Verification items for the finished model (mm, model axes). A direction names the side the tool comes from. Coordinates: 2 decimals unless noted, no trailing zeros. Order: outer loops, then holes, each group sorted by start corner. A loop starts at its lowest first (then second) coordinate and runs counter-clockwise, first axis right, second up. Notation, with made-up numbers: (-23, 14.5) -> (28, 14.5) arc R19 cw to (28, 50.5) -> close; hole circle Ø6 at (-29.75, 62.25). An arc over 180 degrees is marked (long way). Answer as CSV lines item,"result".
Autodesk Inventor part; units mm, degrees
ref_plane "YZ Plane" through (0, 0, 0) normal (1, 0, 0) x (0, 1, 0)
ref_plane "XZ Plane" through (0, 0, 0) normal (0, 1, 0) x (-1, 0, 0)
ref_plane "XY Plane" through (0, 0, 0) normal (0, 0, 1) x (1, 0, 0)
sketch "Sketch1" plane through (0, 0, 0) normal (0, 1, 0) x (-1, 0, 0)
  line L0 (-25, -25) -> (25, -25)
  line L1 (25, -25) -> (25, 25)
  line L2 (25, 25) -> (-25, 25)
  line L3 (-25, 25) -> (-25, -25)
  point P0 (0, 0)
  dimension "d2" = 50
  dimension "d3" = 50
extrude "Extrusion1" add sketch "Sketch1" along normal blind 4
sketch "Sketch2" plane through (0, 4, 0) normal (0, 1, 0) x (1, 0, 0)
  line L0 (-25, 25) -> (-25, -25)
  line L1 (-25, -25) -> (25, -25)
  line L2 (25, -25) -> (25, 25)
  line L3 (25, 25) -> (-25, 25)
  line L4 (-25, -25) -> (25, -25)
  line L5 (0, -25) -> (0, 25)
  line L6 (25, 25) -> (-25, 25)
  line L7 (0, -25) -> (-1.5, -25)
  line L8 (-1.5, -25) -> (1.5, -25)
  line L9 (1.5, -25) -> (1.5, 25)
  line L10 (1.5, 25) -> (-1.5, 25)
  line L11 (-1.5, 25) -> (-1.5, -25)
  line L12 (1.5, 9.2284) -> (-1.5, 9.2284)
  line L13 (1.5, 9.2284) -> (-1.5, 9.2284)
  line L14 (-1.5, 9.2284) -> (-1.5, 25)
  line L15 (-1.5, 25) -> (1.5, 25)
  line L16 (1.5, 25) -> (1.5, 9.2284)
  point P0 (0, 0)
  point P1 (1.5, 25)
  dimension "d6" = 1.5
  dimension "d7" = 3
extrude "Extrusion2" add sketch "Sketch2" along normal blind 3 contours L3 L5 L12 L11 | L3 L9 L12 L5
sketch "Sketch3" plane through (0, 4, 0) normal (0, 1, 0) x (1, 0, 0)
  line L0 (1.5, 25) -> (1.5, 9.2284)
  line L1 (1.5, 9.2284) -> (-1.5, 9.2284)
  line L2 (-1.5, 9.2284) -> (-1.5, 25)
  line L3 (-1.5, 25) -> (-25, 25)
  line L4 (-25, 25) -> (-25, -25)
  line L5 (-25, -25) -> (25, -25)
  line L6 (25, -25) -> (25, 25)
  line L7 (25, 25) -> (1.5, 25)
  line L8 (11.5, 24.5) -> (11.5, 9.7)
  line L9 (-11.5, 9.7) -> (-11.5, 24.5)
  line L10 (25, 25) -> (1.5, 25)
  line L11 (25, 25) -> (11.5, 25)
  line L12 (11.5, 25) -> (11.5, 9.7)
  line L13 (11.5, 9.7) -> (25, 9.7)
  line L14 (25, 9.7) -> (25, 25)
  line L15 (-11.5, 9.7) -> (-25, 9.7)
  line L16 (-25, 9.7) -> (-25, 25)
  line L17 (-25, 25) -> (-11.5, 25)
  line L18 (-11.5, 25) -> (-11.5, 9.7)
  point P0 (0, 0)
extrude "Extrusion3" cut sketch "Sketch3" against normal blind 10 contours L7 L6 L13 L8 L12 | L18 L9 L15 L4 L3
sketch "Sketch4" plane through (0, 0, 0) normal (0, -1, 0) x (1, 0, 0)
  line L0 (-11.5, -9.7) -> (-11.5, -25)
  line L1 (11.5, -25) -> (-11.5, -25)
  line L2 (11.5, -25) -> (11.5, -9.7)
  line L3 (11.5, -9.7) -> (25, -9.7)
  line L4 (25, 25) -> (25, -9.7)
  line L5 (-25, 25) -> (25, 25)
  line L6 (-25, -9.7) -> (-25, 25)
  line L7 (-25, -9.7) -> (-11.5, -9.7)
  point P0 (0, 0)
extrude "Extrusion4" cut sketch "Sketch4" against normal blind 1
sketch "Sketch5" plane through (-25, 4, 25) normal (0, 0, 1) x (1, 0, 0)
  line L0 (0, -3) -> (50, -3)
  line L1 (50, -3) -> (50, 0)
  line L2 (0, 0) -> (50, 0)
  line L3 (0, -3) -> (0, 0)
  line L4 (0, 0) -> (50, 0)
  line L5 (0, 0) -> (50, 0)
  line L6 (50, 0) -> (50, 3)
  line L7 (50, 3) -> (0, 3)
  line L8 (0, 3) -> (0, 0)
  point P0 (25, -4)
  dimension "d14" = 3
extrude "Extrusion5" add sketch "Sketch5" against normal up to surface (34.7 mm away) contours L8 L7 L6 L2
sketch "Sketch6" plane through (11.5, 4, -9.7) normal (0, 0, -1) x (-1, 0, 0)
  line L0 (-13.5, -3) -> (0, -3)
  line L1 (0, 0) -> (0, -3)
  line L2 (10, 0) -> (0, 0)
  line L3 (10, 3) -> (10, 0)
  line L4 (10, 3) -> (-13.5, 3)
  line L5 (-13.5, -3) -> (-13.5, 3)
  line L6 (23, -3) -> (36.5, -3)
  line L7 (36.5, 3) -> (36.5, -3)
  line L8 (36.5, 3) -> (13, 3)
  line L9 (13, 0) -> (13, 3)
  line L10 (23, 0) -> (13, 0)
  line L11 (23, 0) -> (23, -3)
  line L12 (0, 0.5) -> (0, 11.5)
  line L13 (23, 11.5) -> (23, 0.5)
  line L14 (10, 0) -> (0, 0)
  line L15 (0, 11.5) -> (0, 0)
  line L16 (23, 11.5) -> (23, 0)
  line L17 (0, 0) -> (0, -3)
  line L18 (10, 3) -> (-13.5, 3)
  line L19 (0, 0) -> (10, 0)
  line L20 (10, 0) -> (10, 3)
  line L21 (10, 3) -> (0, 3)
  line L22 (0, 3) -> (0, 0)
  line L23 (13, 0) -> (13, 3)
  line L24 (23, 0) -> (23, -3)
  line L25 (13, 3) -> (23, 3)
  line L26 (23, 3) -> (23, 0)
  line L27 (23, 0) -> (13, 0)
  line L28 (13, 0) -> (13, 3)
  point P0 (11.5, -4)
  point P1 (23, 0.5)
  point P2 (0, 3)
extrude "Extrusion6" cut sketch "Sketch6" against normal blind 20 contours L15 L12 L4 L3 L2 | L10 L9 L8 L13 L16
sketch "Sketch7" plane through (11.5, 4, 10.3) normal (0, 0, -1) x (-1, 0, 0)
  arc A0 (0, 2.75) -> (10, 2.7503) centre (4.9999, 5.9206) ccw
  arc A1 (13, 2.75) -> (23, 2.7497) centre (18.0001, 5.9203) ccw
  line L0 (0, 0) -> (10, 0)
  line L1 (5, 0) -> (5, -0.3289)
  line L2 (5, -0.3289) -> (19.1354, -0.3289)
  circle A2 centre (4.9999, 5.9206) radius 6.2495
  circle A3 centre (18.0001, 5.9203) radius 6.2492
  line L3 (0, 3) -> (-13.5, 3)
  line L4 (0, 3) -> (10, 3)
  line L5 (10, 3) -> (10, 0)
  line L6 (10, 0) -> (0, 0)
  line L7 (0, 0) -> (0, 3)
  line L8 (13, 0) -> (13, 3)
  line L9 (23, 3) -> (23, 0)
  line L10 (13, 0) -> (23, 0)
  line L11 (23, 0) -> (23, 3)
  line L12 (23, 3) -> (13, 3)
  line L13 (13, 3) -> (13, 0)
  point P0 (11.5, -4)
  point P1 (20.0008, 0)
  point P2 (23, 2.1715)
  point P3 (15.9994, 0)
  point P4 (13, 2.1717)
  point P5 (10, 2.1715)
  point P6 (7.0007, 0)
  point P7 (0, 2.1713)
  point P8 (2.9992, 0)
extrude "Extrusion7" add sketch "Sketch7" along normal blind 16 contours A2 L0 L7 | A2 L5 L0 | A3 L10 L8 | A3 L9 L10
chamfer "Chamfer1" distance 3 angle 45 2 edges at (6.5, 7, 10.3) (-6.5, 7, 10.3)
sketch "Sketch8" plane through (-25, 7, -9.7) normal (-1, 0, 0) x (0, 0, 1)
  circle A0 centre (-11.34, 3) radius 8
  line L0 (0, -6) -> (34.7, -6)
  line L1 (34.7, -6) -> (34.7, 0)
  line L2 (34.7, 0) -> (0, 0)
  line L3 (0, 0) -> (0, -6)
  line L4 (-11.34, 3) -> (-19.34, 3)
  line L5 (-19.34, 3) -> (-22.34, 3)
  line L6 (-22.34, 3) -> (27.66, 3)
  line L7 (0, -6) -> (34.7, -6)
  line L8 (34.7, -6) -> (27.66, -6)
  line L9 (27.66, -6) -> (27.66, 9.5427)
  line L10 (27.66, 9.5427) -> (34.7, 9.5427)
  line L11 (34.7, 9.5427) -> (34.7, -6)
  point P0 (9.7, -7)
  point P1 (27.66, 0)
  dimension "d24" = 3
  dimension "d25" = 50
extrude "Extrusion8" cut sketch "Sketch8" against normal through all contours L9 L2 L1 L0
sketch "Sketch9" plane through (25, 1, -9.7) normal (1, 0, 0) x (0, 0, -1)
  line L0 (-27.66, 6) -> (-27.66, 0)
  line L1 (-27.66, 0) -> (0, 0)
  line L2 (0, 0) -> (0, 6)
  line L3 (-27.66, 6) -> (0, 6)
  line L4 (-27.66, 0.31) -> (-25.7682, 0.01)
  line L5 (-25.7682, 0.01) -> (-14.0234, 0.01)
  line L6 (-14.0234, 0.01) -> (-14.0234, 0.61)
  line L7 (-25.7682, 0.61) -> (-14.0234, 0.61)
  line L8 (-25.7682, 0.61) -> (-27.66, 0.31)
  line L9 (-27.66, 0) -> (-27.66, 6)
  line L10 (-14.0234, 0.61) -> (-27.66, 0.61)
  line L11 (-27.66, 0.61) -> (-27.66, 1.22)
  line L12 (-27.66, 1.22) -> (-14.0234, 1.22)
  line L13 (-14.0234, 1.22) -> (-14.0234, 0.61)
  point P0 (-9.7, -1)
  point P1 (-27.66, 1.22)
  dimension "d28" = 0.61
extrude "Extrusion9" cut sketch "Sketch9" against normal through all contours L12 L13 L7 L10 L0
sketch "Sketch10" plane through (25, 1, -9.7) normal (1, 0, 0) x (0, 0, -1)
  line L0 (-27.66, 0.31) -> (-25.7682, 0.01)
  line L1 (-25.7682, 0.01) -> (-14.0234, 0.01)
  line L2 (-14.0234, 0.01) -> (-14.0234, 0.61)
  line L3 (-25.7682, 0.61) -> (-14.0234, 0.61)
  line L4 (-25.7682, 0.61) -> (-27.66, 0.31)
  line L5 (-14.0234, 1.22) -> (-14.0234, 0.61)
  line L6 (-27.66, 0) -> (0, 0)
  line L7 (0, 0) -> (0, 6)
  line L8 (-27.66, 6) -> (0, 6)
  line L9 (-27.66, 6) -> (-27.66, 1.22)
  line L10 (-27.66, 1.22) -> (-14.0234, 1.22)
  line L11 (-25.7682, 0.61) -> (-25.7682, 6)
  line L12 (-27.66, 6) -> (0, 6)
  line L13 (-19.9, 5.7) -> (-19.9, 6.1)
  line L14 (15.3, 6) -> (-23, 6)
  line L15 (-19.9, 6) -> (-20.9, 6)
  line L16 (-20.9, 6) -> (-23.9, 6)
  line L17 (-25.7682, 0.61) -> (-23.9, 6)
  line L18 (-14.0234, 0.61) -> (-27.66, 0.61)
  line L19 (-27.66, 0.61) -> (-27.66, 0)
  point P0 (-9.7, -1)
  point P1 (-25.5568, 1.22)
  dimension "d31" = 1
  dimension "d32" = 3
extrude "Extrusion10" cut sketch "Sketch10" against normal through all contours L11 L8 L17 L10 | L10 L9 L8 L11
sketch "Sketch11" plane through (0, 1, 0) normal (0, -1, 0) x (1, 0, 0)
  circle A0 centre (0, -17.35) radius 1.5
  line L0 (3.695, -17.35) -> (1.8475, -14.15)
  line L1 (1.8475, -20.55) -> (3.695, -17.35)
  line L2 (-1.8475, -20.55) -> (1.8475, -20.55)
  line L3 (-3.695, -17.35) -> (-1.8475, -20.55)
  line L4 (-1.8475, -14.15) -> (-3.695, -17.35)
  line L5 (1.8475, -14.15) -> (-1.8475, -14.15)
  circle A1 centre (0, -17.35) radius 1.5
  line L6 (-25, -10.04) -> (-25, -32.04)
  point P0 (0, 0)
extrude "Extrusion11" cut sketch "Sketch11" against normal through all contours A0
chamfer "Chamfer2" distance 1 angle 45 1 edges at (-1.5, 1, -17.35)
sketch "Sketch12" plane through (-25, 1, -9.7) normal (-1, 0, 0) x (0, 0, 1)
  line L0 (25.5568, 1.22) -> (23.9, 6)
  line L1 (23.9, 6) -> (0, 6)
  line L2 (0, 6) -> (0, 0)
  line L3 (0, 0) -> (27.66, 0)
  line L4 (27.66, 0) -> (27.66, 0.61)
  line L5 (27.66, 0.61) -> (14.0234, 0.61)
  line L6 (14.0234, 0.61) -> (14.0234, 1.22)
  line L7 (14.0234, 1.22) -> (25.5568, 1.22)
  circle A0 centre (-11.34, 9) radius 11
  line L8 (-22.34, 9) -> (27.66, 9)
  line L9 (27.66, 9) -> (27.66, -12.93)
  line L10 (-11.34, 9) -> (-11.34, -2)
  line L11 (-11.34, -2) -> (27.66, -1.965)
  line L12 (14.0234, 1.22) -> (25.5568, 1.22)
  line L13 (27.66, -1.3745) -> (14.0234, 1.22)
  line L14 (14.0234, 1.22) -> (14.0795, 1.5147)
  line L15 (14.0234, 1.22) -> (13.9673, 0.9253)
  line L16 (14.0795, 1.5147) -> (28.9229, -1.3094)
  line L17 (13.9673, 0.9253) -> (29.035, -1.9638)
  line L18 (25.5568, 1.22) -> (24.566, 4.0785)
  line L19 (25.5568, 1.22) -> (23.9, 6)
  line L20 (25.5568, 1.22) -> (26.2577, -0.8023)
  point P0 (9.7, -1)
  point P1 (15.6117, 0.61)
  point P2 (14.0234, 0.9145)
  point P3 (15.6285, 1.22)
  dimension "d40" = 0.3
  dimension "d41" = 0.3
extrude "Extrusion12" add sketch "Sketch12" against normal blind 50 contours L20 L5 L16 L7 | L20 L3 L16 L5 | L20 L16 L3 | L17 L5 L6
sketch "Sketch13" plane through (-25, 1, -9.7) normal (-1, 0, 0) x (0, 0, 1)
  line L0 (18.8347, 0.61) -> (15.6117, 0.61)
  line L1 (15.6117, 0.61) -> (14.0234, 0.9145)
  line L2 (14.0234, 0.9145) -> (14.0234, 1.22)
  line L3 (14.0234, 1.22) -> (15.6285, 1.22)
  line L4 (15.6285, 1.22) -> (18.8347, 0.61)
  line L5 (25.7682, 0.61) -> (23.9, 6)
  line L6 (23.9, 6) -> (0, 6)
  line L7 (0, 6) -> (0, 0)
  line L8 (0, 0) -> (22.0408, 0)
  line L9 (22.0408, 0) -> (26.2577, -0.8023)
  line L10 (26.2577, -0.8023) -> (25.9796, 0)
  line L11 (25.9796, 0) -> (27.66, 0)
  line L12 (27.66, 0) -> (27.66, 0.61)
  line L13 (27.66, 0.61) -> (25.7682, 0.61)
  line L14 (14.0234, 0.9145) -> (14.0234, 1.22)
  line L15 (14.0234, 0.9145) -> (26.7141, -1.5188)
  line L16 (14.0234, 1.22) -> (15.6285, 1.22)
  line L17 (15.6285, 1.22) -> (29.31, -1.383)
  line L18 (14.0234, 0.9145) -> (13.2268, 1.0673)
  line L19 (13.2268, 1.0673) -> (13.3704, 1.8159)
  line L20 (15.6285, 1.22) -> (13.3396, 1.6555)
  line L21 (25.9796, 0) -> (27.66, 0)
  line L22 (25.9796, 0) -> (25.7682, 0.61)
  line L23 (26.7141, -1.5188) -> (27.0047, -0.9444)
  point P0 (9.7, -1)
  point P1 (18.7931, 0)
extrude "Extrusion13" cut sketch "Sketch13" against normal through all contours L17 L8 L15 L0 | L3 L2 L18 L19 L20 | L22 L13 L12 L11
sketch "Sketch14" plane through (-25, 1, -9.7) normal (-1, 0, 0) x (0, 0, 1)
  line L0 (26.2577, -0.8023) -> (23.9, 6)
  line L1 (23.9, 6) -> (0, 6)
  line L2 (0, 6) -> (0, 0)
  line L3 (0, 0) -> (18.7931, 0)
  line L4 (18.7931, 0) -> (13.2268, 1.0673)
  line L5 (13.2268, 1.0673) -> (13.3396, 1.6555)
  line L6 (13.3396, 1.6555) -> (26.2577, -0.8023)
  circle A0 centre (-11.34, 9) radius 11
  line L7 (-22.34, 9) -> (27.66, 9)
  line L8 (-11.34, 9) -> (-11.34, -2)
  line L9 (-11.34, 9) -> (27.66, 9)
  line L10 (27.66, 9) -> (27.66, -2)
  line L11 (27.66, -2) -> (-11.34, -2)
  line L12 (-11.34, -2) -> (-11.34, 9)
  line L13 (4, 3) -> (-7.65, 3)
  line L14 (-7.65, 3) -> (-15.3, 3)
  line L15 (-15.3, 3) -> (0, 3)
  line L16 (0, 3) -> (4, 3)
  line L17 (4, 3) -> (20, 3)
  line L18 (20, 3) -> (4, 3)
  line L19 (0, 3) -> (-15.3, 3)
  line L20 (0, 3) -> (20, 3)
  line L21 (20, 3) -> (20, 2)
  line L22 (20, 2) -> (0, 2)
  line L23 (0, 2) -> (0, 3)
  line L24 (22.1715, 5.1715) -> (20, 3)
  line L25 (20, 3) -> (29.0462, 3)
  line L26 (29.0462, 3) -> (29.0462, 2)
  line L27 (29.0462, 2) -> (20, 2)
  line L28 (20, 2) -> (20, 3)
  line L29 (27.66, 2) -> (-2.34, 2)
  line L30 (-2.34, 2) -> (-2.34, -1)
  line L31 (-2.34, -1) -> (27.66, -1)
  line L32 (27.66, -1) -> (27.66, 2)
  line L33 (27.66, -1) -> (24.0847, 2)
  line L34 (26.2577, -0.8023) -> (23.9, 6)
  line L35 (24.0847, 2) -> (23.5108, 6)
  line L36 (23.9, 6) -> (0, 6)
  point P0 (9.7, -1)
  point P1 (24.0847, 2)
  point P2 (25.7792, 0.5781)
  dimension "d46" = 50
  dimension "d47" = 1
  dimension "d48" = 30
  dimension "d49" = 3
  dimension "d50" = 40
extrude "Extrusion14" cut sketch "Sketch14" against normal through all contours L6 L5 L4 L3 L2 L22 L27 L33 L0 | L0 L33 L31 L30 L29 L2 L3 L4 L5 L6 | L33 L27 L0 | L27 L35 L25 L0 | L25 L35 L1 L0
properties part number "podsta"
Item 1: Tool access check on faces 4 (the flat face through (0, 3, 1)), 5 (the flat face through (-18, 5, -9.7)), 6 (the flat face through (18, 5, -9.7)), 7 (the cylindrical face through (-10.186, 4.874, 3.513)). Record the directions out of +Z, -Z, +X, -X, +Y, -Y that give a thin tool (end or side, any length) a straight path to the whole face; none if there is none.
Answer list:
face 4,"+Z, +X, -X, -Y"
face 5,"-Z, -X, +Y, -Y"
face 6,"-Z, +X, +Y, -Y"
face 7,"-Z, +Y"
Item 2: Release check for a two-part mould opening along X. For faces 1 (the cylindrical face through (-2.86, 4.84, 3.51)), 2 (the flat face through (-3, 1, -18)), 3 (the flat face through (1.5, 5, -21)) record: +X half, -X half, draft (parallel to the pull), parting line (faces both ways), or undercut.
Answer list:
face 1,"undercut"
face 2,"draft"
face 3,"+X half"
Item 3: Section check A-A, the plane x = 0. Record the boundary of the cut face in (y, z).
Answer list:
outline,"(1, -25) -> (7, -25) -> (7, -18.85) -> (2, -18.85) -> (1, -19.85) -> close; (1, -14.85) -> (2, -15.85) -> (7, -15.85) -> (7, 13.81) -> (3, 14.38) -> (3, -12.04) -> (1, -12.04) -> close"
Item 4: Section check C-C, the plane x = -16.5. Record the boundary of the cut face in (y, z), plus the area to 3 significant figures.
Answer list:
outline,"(3, -9.7) -> (7, -9.7) -> (7, 13.81) -> (3, 14.38) -> close"
area,"95.2 mm2"
Item 5: Depth check by flat-ended pin: pin 1 Ø3 at (x, y) = (18, 5.5) entering from -Z; pin 2 Ø2.5 at (y, z) = (5, -23) entering from +X; pin 3 Ø1.5 at (x, z) = (-7.5, 10) entering from +Y; pin 4 Ø2.5 at (x, z) = (0, -17.35) entering from +Y. Enter the tip coordinate at first touch or a pass-through.
Answer list:
pin 1,"z = -9.7"
pin 2,"x = 11.5"
pin 3,"y = 4.45"
pin 4,"through"
Item 6: Thickness scan on line 1 (Y direction, x = -15, z = -3); line 2 (X direction, y = 5.75, z = 3.5); line 3 (X direction, y = 1.75, z = -22). Record the ranges inside material, lowest first.
Answer list:
line 1,"3 to 7"
line 2,"-25 to -11.15, -1.85 to 1.85, 11.15 to 25"
line 3,"-11.5 to 11.5"
Item 7: Section check B-B, the plane z = 8.5. Record the boundary of the cut face in (x, y).
Answer list:
outline,"(-25, 3) -> (25, 3) -> (25, 7) -> (11.5, 7) -> (11.5, 6.17) arc R6.25 cw to (8.5, 4) -> (4.5, 4) arc R6.25 cw to (1.5, 6.17) -> (1.5, 7) -> (-1.5, 7) -> (-1.5, 6.17) arc R6.25 cw to (-4.5, 4) -> (-8.5, 4) arc R6.25 cw to (-11.5, 6.17) -> (-11.5, 7) -> (-25, 7) -> close"
